from build123d import *

# Parameters (mm, degrees)
SKETCH3_R           = 1.6
BOSS_EXTRUDE1_DEPTH = 5
SKETCH4_W           = 13.182571809
SKETCH4_H           = 60
CUT_EXTRUDE1_DEPTH  = 1
FILLET1_R           = 5
FILLET2_R           = 3


with BuildPart() as part:
    # Sketch3 → Boss-Extrude1 (new body, symmetric)
    with BuildSketch(Plane(origin=(0, 0, 0), x_dir=(1, 0, 0), z_dir=(0, 1, 0))):
        Polygon((-81.692561237, 30), (-81.692561237, 26.25), (-85, 22.942561237), (-85, -22.942561237), (-81.692561237, -26.25), (-81.692561237, -30), (-81.692561237, -35), (-93.75, -35), (-93.75, 35), (-81.692561237, 35), align=None)
        with Locations((-85, 26.25)):
            Circle(SKETCH3_R, mode=Mode.SUBTRACT)
        with Locations((-85, -26.25)):
            Circle(SKETCH3_R, mode=Mode.SUBTRACT)
    extrude(amount=BOSS_EXTRUDE1_DEPTH, both=True)

    # Sketch4 → Cut-Extrude1 (cut, symmetric)
    with BuildSketch(Plane(origin=(0, 0, 0), x_dir=(1, 0, 0), z_dir=(0, 1, 0))):
        with Locations((-82.158714096, 0)):
            Rectangle(SKETCH4_W, SKETCH4_H)
    extrude(amount=CUT_EXTRUDE1_DEPTH, both=True, mode=Mode.SUBTRACT)

    # Fillet1
    fillet1_edges = [part.edges().sort_by_distance(p)[0] for p in [
        (-81.692561237, 3, -26.25),
        (-85, 3, -22.942561237),
        (-85, 3, 22.942561237),
        (-81.692561237, 3, 26.25),
        (-81.692561237, -3, -26.25),
        (-85, -3, -22.942561237),
        (-85, -3, 22.942561237),
        (-81.692561237, -3, 26.25),
    ]]
    fillet(fillet1_edges, radius=FILLET1_R)

    # Fillet2
    fillet2_edges = [part.edges().sort_by_distance(p)[0] for p in [
        (-81.692561237, 0, 35),
        (-93.75, 0, 35),
        (-93.75, 0, -35),
        (-81.692561237, 0, -35),
    ]]
    fillet(fillet2_edges, radius=FILLET2_R)


solid = part.part
Part model, mm, in its own coordinate system. A direction names the side the tool comes from. Round coordinates to 2 decimals unless told otherwise and drop trailing zeros. Loops run counter-clockwise (first coordinate to the right, second up) from the corner with the lowest first, then second, coordinate; pieces in that order, holes last. Notation, with made-up numbers: (79, -31.5) - (111, -31.5) arc R10 ccw to (111, -21.5) - close; hole circle Ø4 at (57, 19.5). An arc over 180 degrees is marked (long way). Answer as a JSON object with one key per item and string values.
Item 1: Tool access for faces 5 (the face through (-82.063, 2.972, -26.433)), 6 (the face through (-85, 0, -30)), 7 (the face through (-92.89, 0.07, 34.1)): list every direction of +Z, -Z, +X, -X, +Y, -Y with a clear straight run to the whole face (end or side of a thin tool).
Output:
{"face 5": "+X, +Y, -Y", "face 6": "+X", "face 7": "+Z, -X, +Y, -Y"}
Item 2: Pull direction Z, two halves, no side cores. Call faces 1 (the face through (-82.55, 0.07, -34.1)), 2 (the face through (-89, 5, 0)), 3 (the face through (-86.6, -3, 26.2)), 4 (the face through (-82.063, -3.028, -26.433)): pulls with the +Z half, pulls with the -Z half, needs draft (parallel to the pull), parting line crosses it, or undercut.
Output:
{"face 1": "pulls with the -Z half", "face 2": "needs draft", "face 3": "undercut", "face 4": "undercut"}
Item 3: Wall check: L1, parallel to Y at x = -87.25, z = 3.5; L2, parallel to X at y = 0.75, z = -17.5; L3, parallel to X at y = 1.75, z = 17.5. Give the ranges that are in metal, low to high.
Output:
{"L1": "-5 to -1, 1 to 5", "L2": "-93.75 to -88.75", "L3": "-93.75 to -85"}
Item 4: Pin check, flat tips, straight feed: pin 1 (1.2 mm diameter, centred on y = -2, z = 9.5, fed in from +X); pin 2 (0.6 mm diameter, centred on y = 0.5, z = 2, fed in from +X). Stop position of each tip, or through.
Output:
{"pin 1": "x = -85", "pin 2": "x = -88.75"}
Item 5: Band-saw the part on C-C on z = 26.25. List the corners of the cut face in (x, y), plus the area to 3 significant figures.
Output:
{"outline": "(-93.75, -5) - (-86.6, -5) - (-86.6, -1) - (-88.75, -1) - (-88.75, 1) - (-86.6, 1) - (-86.6, 5) - (-93.75, 5) - close; (-83.4, -5) - (-82.14, -5) - (-82.14, -1) - (-83.4, -1) - close; (-83.4, 1) - (-82.14, 1) - (-82.14, 5) - (-83.4, 5) - close", "area": "77.3 mm2"}
Item 6: Band-saw the part on B-B on z = -18. List the corners of the cut face in (x, y), plus the area to 3 significant figures.
Output:
{"outline": "(-93.75, -5) - (-85, -5) - (-85, -1) - (-88.75, -1) - (-88.75, 1) - (-85, 1) - (-85, 5) - (-93.75, 5) - close", "area": "80.0 mm2"}
Item 7: Band-saw the part on A-A on y = 4. List the corners of the cut face in (x, z), plus the area to 3 significant figures.
Output:
{"outline": "(-93.75, -32) arc R3 ccw to (-90.75, -35) - (-84.69, -35) arc R3 ccw to (-81.69, -32) - (-81.69, -28.32) arc R5 ccw to (-83.16, -24.79) - (-83.54, -24.41) arc R5 cw to (-85, -20.87) - (-85, 20.87) arc R5 cw to (-83.54, 24.41) - (-83.16, 24.79) arc R5 ccw to (-81.69, 28.32) - (-81.69, 32) arc R3 ccw to (-84.69, 35) - (-90.75, 35) arc R3 ccw to (-93.75, 32) - close; hole circle Ø3.2 at (-85, -26.25); hole circle Ø3.2 at (-85, 26.25)", "area": "658 mm2"}
